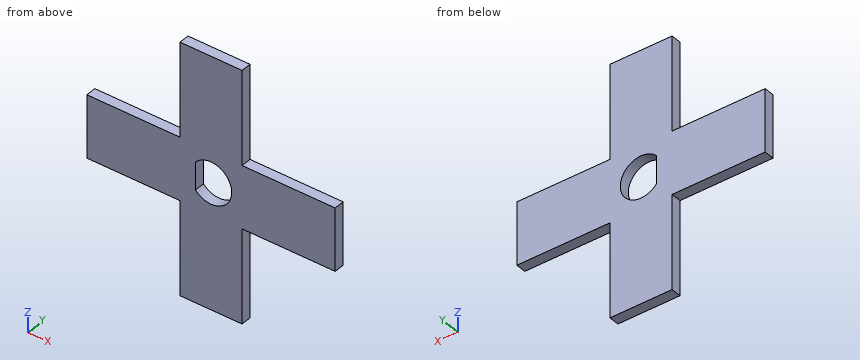
from build123d import *

# Parameters (mm, degrees)
BOSS_EXTRUDE1_DEPTH = 2
CUT_EXTRUDE2_DEPTH  = 35


with BuildPart() as part:
    # Sketch1 → Boss-Extrude1 (new body)
    with BuildSketch(Plane(origin=(0, 0, 0), x_dir=(1, 0, 0), z_dir=(0, 1, 0))):
        Polygon((-6, 6), (-6, 24), (6, 24), (6, 6), (24, 6), (24, -6), (6, -6), (6, -24), (-6, -24), (-6, -6), (-24, -6), (-24, 6), align=None)
    extrude(amount=BOSS_EXTRUDE1_DEPTH)

    # Sketch2 → Cut-Extrude2 (cut, through all)
    with BuildSketch(Plane(origin=(0, 0, 0), x_dir=(1, 0, 0), z_dir=(0, 1, 0))):
        with BuildLine():
            Line((-3, -2.645751311), (-3, 2.645751311))
            ThreePointArc((-3, 2.645751311), (4, 0), (-3, -2.645751311))
        make_face()
    extrude(amount=CUT_EXTRUDE2_DEPTH, mode=Mode.SUBTRACT)


solid = part.part
CAD build for the part. Positions are in the model's coordinates, mm. Give positions to 0.01 mm unless a question says otherwise; leave off trailing zeros. Loops run counter-clockwise (first coordinate to the right, second up) from the corner with the lowest first, then second, coordinate; pieces in that order, holes last. Notation, with made-up numbers: M 80.25,21 L 96.25,21 A27 cw 96.25,47 Z; hole C 10.25,72.5 d5. An arc over 180 degrees is marked long. Answer in a Markdown table with one row per item. Add a question column.
Item 1: Band-saw the part on B-B on z = 0. Give the cut face in (x, y), then the cut area to 3 significant figures.
Item 2: Drop flat-ended pins along their axis: P1, Ø1, axis at y = 1, z = 11.5, coming from the -X side; P2, Ø1, axis at x = 11.5, y = 0.5, coming from the -Z side; P3, Ø0.6, axis at y = 1.5, z = 16, coming from the +X side. Give the stop position or say it passes through.
Item 3: Band-saw the part on A-A on x = 0. Give the cut face in (y, z), then the cut area to 3 significant figures.
Item 4: Probe probe 1 along X at (y, z) = (0.55, 0); probe 2 along Z at (x, y) = (0, 0.55); probe 3 along X at (y, z) = (1.4, 19.5). List the from-to ranges inside material, lowest first.
Item 5: Band-saw the part on C-C on y = 1. Give the cut face in (x, z).
Item 6: Band-saw the part on D-D on z = 15. Give the cut face in (x, y).
Reply:
| question | item | result |
|---|---|---|
| 1 | outline | M -24,0 L -3,0 L -3,2 L -24,2 Z; M 4,0 L 24,0 L 24,2 L 4,2 Z |
| 1 | area | 82.0 mm^2 |
| 2 | P1 | stops at x = -6 |
| 2 | P2 | stops at z = -6 |
| 2 | P3 | stops at x = 6 |
| 3 | outline | M 0,-24 L 2,-24 L 2,-4 L 0,-4 Z; M 0,4 L 2,4 L 2,24 L 0,24 Z |
| 3 | area | 80.0 mm^2 |
| 4 | probe 1 | x = -24 to -3, 4 to 24 |
| 4 | probe 2 | z = -24 to -4, 4 to 24 |
| 4 | probe 3 | x = -6 to 6 |
| 5 | outline | M -24,-6 L -6,-6 L -6,-24 L 6,-24 L 6,-6 L 24,-6 L 24,6 L 6,6 L 6,24 L -6,24 L -6,6 L -24,6 Z; hole M -3,-2.65 A4 ccw long -3,2.65 Z |
| 6 | outline | M -6,0 L 6,0 L 6,2 L -6,2 Z |
